```python
from build123d import *

# Parameters (mm, degrees)
SKETCH2_R               = 105
BOSS_EXTRUDE1_DEPTH     = 3.625
CUT_EXTRUDE1_DEPTH      = 184.813392126
CUT_EXTRUDE1_DEPTH_BACK = 184.813392126
SKETCH4_R               = 1.25
SKETCH7_R               = 1.05
CUT_EXTRUDE2_DEPTH      = 184.920594346
CUT_EXTRUDE3_DEPTH      = 184.813392191
CUT_EXTRUDE3_DEPTH_BACK = 184.813392191
SKETCH9_R               = 1.05
CUT_EXTRUDE4_DEPTH      = 184.813392192
CUT_EXTRUDE4_DEPTH_BACK = 184.813392192
SKETCH10_W              = 20
SKETCH10_H              = 10
CUT_EXTRUDE5_DEPTH      = 184.745375857
CUT_EXTRUDE5_DEPTH_BACK = 184.745375857
SKETCH11_W              = 30
SKETCH11_H              = 90
SKETCH12_R              = 1.05
CUT_EXTRUDE6_DEPTH      = 7.25
FILLET1_R               = 1
SKETCH13_W              = 130
SKETCH13_H              = 10
CUT_EXTRUDE7_DEPTH      = 1
FILLET2_R               = 2


with BuildPart() as part:
    # Sketch2 → Boss-Extrude1 (new, symmetric)
    with BuildSketch(Plane(origin=(0, 0, 0), x_dir=(1, 0, 0), z_dir=(0, 1, 0))):
        with BuildLine():
            Line((-33, -135), (-33, -143.35))
            Line((-33, -143.35), (-21, -143.35))
            Line((-21, -143.35), (-21, -135))
            ThreePointArc((-21, -135), (-22.264456843, -123.242302365), (-26, -112.022319205))
            ThreePointArc((-26, -112.022319205), (0, -115), (26, -112.022319205))
            ThreePointArc((26, -112.022319205), (22.264456843, -123.242302365), (21, -135))
            Line((21, -135), (21, -143.35))
            Line((21, -143.35), (33, -143.35))
            Line((33, -143.35), (33, -135))
            ThreePointArc((33, -135), (35.810957179, -119.65357728), (43.878842197, -106.299798718))
            ThreePointArc((43.878842197, -106.299798718), (0, 115), (-43.878842197, -106.299798718))
            ThreePointArc((-43.878842197, -106.299798718), (-35.810957179, -119.65357728), (-33, -135))
        make_face()
        with Locations(Location((0, 0, 0), (0, 0, 90))):
            Circle(SKETCH2_R, mode=Mode.SUBTRACT)
    extrude(amount=BOSS_EXTRUDE1_DEPTH, both=True)

    # Sketch4 → Cut-Extrude1 (cut, two sides: drawn at the far end of the back side and taken through both)
    with BuildSketch(Plane(origin=(0, 0, 0), x_dir=(0, 1, 0), z_dir=(0.39874906892524387, 0, -0.9170600743851252)).offset(-CUT_EXTRUDE1_DEPTH_BACK)):
        with Locations(Location((0, 0, 0), (0, 0, 270))):
            Circle(SKETCH4_R)
    extrude(amount=CUT_EXTRUDE1_DEPTH + CUT_EXTRUDE1_DEPTH_BACK, mode=Mode.SUBTRACT)

    # Sketch7 → Cut-Extrude2 (cut, through all)
    with BuildSketch(Plane(origin=(0, 3.625, 0), x_dir=(1, 0, 0), z_dir=(0, 1, 0))):
        with Locations(Location((-30, -141, 0), (0, 0, 270))):
            Circle(SKETCH7_R)
        with Locations(Location((-24, -141, 0), (0, 0, 270))):
            Circle(SKETCH7_R)
        with Locations(Location((24, -141, 0), (0, 0, 270))):
            Circle(SKETCH7_R)
        with Locations(Location((30, -141, 0), (0, 0, 270))):
            Circle(SKETCH7_R)
    extrude(amount=-CUT_EXTRUDE2_DEPTH, mode=Mode.SUBTRACT)

    # Sketch9 → Cut-Extrude3 (cut, two sides: drawn at the far end of the back side and taken through both)
    with BuildSketch(Plane(origin=(0, 0, 0), x_dir=(0, 0, -1), z_dir=(1, 0, 0)).offset(-CUT_EXTRUDE3_DEPTH_BACK)):
        with Locations(Location((0, 0, 0), (0, 0, 180))):
            Circle(SKETCH9_R)
    extrude(amount=CUT_EXTRUDE3_DEPTH + CUT_EXTRUDE3_DEPTH_BACK, mode=Mode.SUBTRACT)

    # Sketch10 → Cut-Extrude4 (cut, two sides: drawn at the far end of the back side and taken through both)
    with BuildSketch(Plane(origin=(0, 0, 0), x_dir=(1, 0, 0), z_dir=(0, 1, 0)).offset(-CUT_EXTRUDE4_DEPTH_BACK)):
        with Locations((-120, 0)):
            Rectangle(SKETCH10_W, SKETCH10_H)
        with Locations((120, 0)):
            Rectangle(SKETCH10_W, SKETCH10_H)
    extrude(amount=CUT_EXTRUDE4_DEPTH + CUT_EXTRUDE4_DEPTH_BACK, mode=Mode.SUBTRACT)

    # Sketch11 → Cut-Extrude5 (cut, two sides: drawn at the far end of the back side and taken through both)
    with BuildSketch(Plane(origin=(0, 0, 0), x_dir=(1, 0, 0), z_dir=(0, 1, 0)).offset(-CUT_EXTRUDE5_DEPTH_BACK)):
        with Locations((-127.391252931, 0)):
            Rectangle(SKETCH11_W, SKETCH11_H)
        with Locations((127.391252931, 0)):
            Rectangle(SKETCH11_W, SKETCH11_H)
    extrude(amount=CUT_EXTRUDE5_DEPTH + CUT_EXTRUDE5_DEPTH_BACK, mode=Mode.SUBTRACT)

    # Sketch12 → Cut-Extrude6 (cut)
    with BuildSketch(Plane(origin=(0, 3.625, 0), x_dir=(1, 0, 0), z_dir=(0, 1, 0))):
        with Locations(Location((0, -107.45, 0), (0, 0, 270))):
            Circle(SKETCH12_R)
    extrude(amount=-CUT_EXTRUDE6_DEPTH, mode=Mode.SUBTRACT)

    # Fillet1
    fillet1_edges = [part.edges().sort_by_distance(p)[0] for p in [
        (-27, -3.625, 143.35),
        (27, -3.625, 143.35),
        (-21, 0, 143.35),
        (-33, 0, 143.35),
        (27, 3.625, 143.35),
        (33, 0, 143.35),
        (21, 0, 143.35),
        (-27, 3.625, 143.35),
    ]]
    fillet(fillet1_edges, radius=FILLET1_R)

    # Sketch13 → Cut-Extrude7 (cut)
    with BuildSketch(Plane(origin=(0, 3.625, 0), x_dir=(1, 0, 0), z_dir=(0, 1, 0))):
        with Locations((0, -140)):
            Rectangle(SKETCH13_W, SKETCH13_H)
    extrude(amount=-CUT_EXTRUDE7_DEPTH, mode=Mode.SUBTRACT)

    # Fillet2
    # the kernel refuses this fillet: 2 mm, written as the material it takes off along each edge
    with BuildSketch(Plane(origin=(37.330127019, 3.625, 135), x_dir=(0, 0, -1), z_dir=(-1, 0, 0))) as fillet2_piece_1:
        with BuildLine():
            CenterArc((1.732050808, 2), FILLET2_R, 210, 60)
            Line((0, 1), (-0.034641016, 0.98))
            ThreePointArc((-0.034641016, 0.98), (-0.04, 0.5), (-0.04, 0))
            Line((-0.04, 0), (0, -0.04))
            Line((0, -0.04), (1.732050808, -0.04))
            Line((1.732050808, -0.04), (1.732050808, 0))
        make_face()
    extrude(amount=20.660254038, mode=Mode.SUBTRACT)
    with BuildSketch(Plane(origin=(-16.669872981, 3.625, 135), x_dir=(0, -1, 0), z_dir=(-1, 0, 0))) as fillet2_piece_2:
        with BuildLine():
            CenterArc((2, -1.732050808), FILLET2_R, 120, 60)
            Line((0, -1.732050808), (-0.04, -1.732050808))
            Line((-0.04, -1.732050808), (-0.04, 0))
            Line((-0.04, 0), (0, 0.04))
            ThreePointArc((0, 0.04), (0.5, 0.04), (0.98, 0.034641016))
            Line((0.98, 0.034641016), (1, 0))
        make_face()
    extrude(amount=20.660254038, mode=Mode.SUBTRACT)


solid = part.part
```
The listing builds one solid part. Answer for the finished solid, in the listing's coordinates (mm). A direction names the side the tool comes from. Give positions to 0.01 mm unless a question says otherwise; leave off trailing zeros. Order: outer loops, then holes, each group sorted by start corner. A loop starts at its lowest first (then second) coordinate and runs counter-clockwise, first axis right, second up. Notation, with made-up numbers: (83.25, 30) -> (141.25, 30) arc R16 cw to (141.25, 48) -> close; hole circle Ø4 at (4.25, 41). An arc over 180 degrees is marked (long way). Write each question's results on one line, items separated by ' | '.
Q1. Determine the mould class of faces 4 (the face through (-22.23, 0.05, 123.4)), 5 (the face through (-42, -3.625, 99)), 6 (the face through (2.19, 0.05, -114.98)), 7 (the face through (27, 0, 143.35)) for opening direction Z: pulls with the +Z half, pulls with the -Z half, needs draft (parallel to the pull), parting line crosses it, or undercut.
Checked values:
face 4: undercut | face 5: needs draft | face 6: pulls with the -Z half | face 7: pulls with the +Z half
Q2. The part is cut by section B-B, the plane x = -57. Give the vertices of the cut face in (y, z) (3 decimals).
Checked values:
outline: (-3.625, -99.88) -> (3.625, -99.88) -> (3.625, -88.182) -> (-3.625, -88.182) -> close; (-3.625, 88.182) -> (3.625, 88.182) -> (3.625, 99.88) -> (-3.625, 99.88) -> close
Q3. The part is cut by section A-A, the plane z = 29. Give the vertices of the cut face in (x, y) (3 decimals), and give its area (3 significant figures).
Checked values:
outline: (-111.283, -3.625) -> (-100.916, -3.625) -> (-100.916, 3.625) -> (-111.283, 3.625) -> close; (100.916, -3.625) -> (111.283, -3.625) -> (111.283, 3.625) -> (100.916, 3.625) -> close | area: 150 mm^2
Q4. Each of these flat-tipped pins is pushed along its axis until it touches: P1, Ø2.5, axis at x = 24, z = 141, coming from the +Y side (3 decimals); P2, Ø1, axis at y = 1.5, z = 46, coming from the +X side; P3, Ø3, axis at x = 18.5, y = 1, coming from the +Z side. Where does it stop, or does it pass through?
Checked values:
P1: stops at y = 2.625 | P2: stops at x = 105.62 | P3: stops at z = 113.74
Q5. Straight lines are drawn through the part: probe 1 along X at (y, z) = (0, 141); probe 2 along Y at (x, z) = (106.7, 0) (3 decimals); probe 3 along X at (y, z) = (2, -96). For each, find the intervals that lie inside material, in ascending order. Write a range as from..to.
Checked values:
probe 1: x = -33..-31.05, -28.95..-25.05, -22.95..-21, 21..22.95, 25.05..28.95, 31.05..33 | probe 2: y = -3.625..-1.05, 1.05..3.625 | probe 3: x = -63.32..-42.53, 42.53..63.32
Q6. Which of the six approach directions +Z, -Z, +X, -X, +Y, -Y give full straight-line access (tool end or side, diameter ignored) to faces 1 (the face through (-33, 0, 139)), 2 (the face through (21, 0, 139)), 3 (the face through (-27, 2.625, 139))?
Checked values:
face 1: +Z, -X, +Y, -Y | face 2: +Z, +Y, -Y | face 3: +Z, +X, -X, +Y
